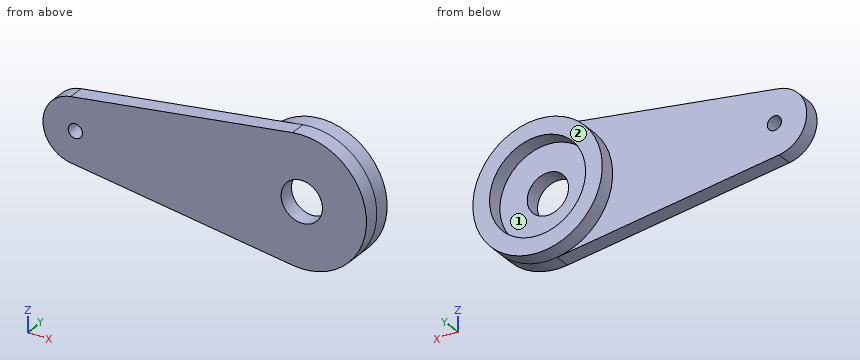
from build123d import *
from build123d.topology import SkipClean

# Parameters (mm, degrees)
EXTRUDE1_DEPTH                      = 6.35
EXTRUDE2_START                      = 6.35
SKETCH2_R                           = 25.4
EXTRUDE2_DEPTH                      = 6.35
F_7_32_0_21875_DIAMETER_HOLE1_D     = 5.55625
F_7_32_0_21875_DIAMETER_HOLE1_DEPTH = 25.4
F_7_32_0_21875_DIAMETER_HOLE1_TIP   = 1.669265907
SKETCH5_R                           = 18.848677946
EXTRUDE3_DEPTH                      = 6.35
SKETCH6_R                           = 8.113502116
EXTRUDE5_DEPTH                      = 118.260276735


with BuildPart() as part:
    # Sketch1 → Extrude1 (new body)
    with BuildSketch(Plane(origin=(0, 0, 0), x_dir=(1, 0, 0), z_dir=(0, 1, 0))):
        with BuildLine():
            Line((-1.814285714, 12.569740146), (85.271428571, 25.139480293))
            ThreePointArc((85.271428571, 25.139480293), (114.3, 0), (85.271428571, -25.139480293))
            Line((85.271428571, -25.139480293), (-1.814285714, -12.569740146))
            ThreePointArc((-1.814285714, -12.569740146), (-12.7, 0), (-1.814285714, 12.569740146))
        make_face()
    extrude(amount=-EXTRUDE1_DEPTH)

    # Sketch2 → Extrude2 (add)
    with SkipClean():  # the faces are left unmerged after this step: merging them gives an invalid solid
        with BuildSketch(Plane(origin=(0, 0, 0), x_dir=(1, 0, 0), z_dir=(0, 1, 0)).offset(EXTRUDE2_START)):
            with Locations(Location((88.9, 0, 0), (0, 0, 270))):
                Circle(SKETCH2_R)
        extrude(amount=-EXTRUDE2_DEPTH)

    # 7/32 (0.21875) Diameter Hole1
    with Locations(Plane.ZX):
        with Locations((0, 0)):
            Hole(F_7_32_0_21875_DIAMETER_HOLE1_D / 2, depth=F_7_32_0_21875_DIAMETER_HOLE1_DEPTH)
            with Locations((0, 0, -(F_7_32_0_21875_DIAMETER_HOLE1_DEPTH + F_7_32_0_21875_DIAMETER_HOLE1_TIP / 2))):  # 118° drill point
                Cone(0, F_7_32_0_21875_DIAMETER_HOLE1_D / 2, F_7_32_0_21875_DIAMETER_HOLE1_TIP, mode=Mode.SUBTRACT)

    # Sketch5 → Extrude3 (cut)
    with SkipClean():  # the faces are left unmerged after this step: merging them gives an invalid solid
        with BuildSketch(Plane(origin=(0, 6.35, 0), x_dir=(-1, 0, 0), z_dir=(0, 1, 0))):
            with Locations(Location((-88.9, 0, 0), (0, 0, 90))):
                Circle(SKETCH5_R)
        extrude(amount=-EXTRUDE3_DEPTH, mode=Mode.SUBTRACT)

    # Sketch6 → Extrude5 (cut, through all)
    with SkipClean():  # the faces are left unmerged after this step: merging them gives an invalid solid
        with BuildSketch(Plane(origin=(0, 0, 0), x_dir=(-1, 0, 0), z_dir=(0, 1, 0))):
            with Locations(Location((-88.9, 0, 0), (0, 0, 90))):
                Circle(SKETCH6_R)
        extrude(amount=-EXTRUDE5_DEPTH, mode=Mode.SUBTRACT)


solid = part.part
Input: part model. Units: mm. Frame: model coordinates. Face numbers are marked on the shaded views. Give positions to 0.01 mm unless a question says otherwise; leave off trailing zeros. Order: outer loops, then holes, each group sorted by start corner. A loop starts at its lowest first (then second) coordinate and runs counter-clockwise, first axis right, second up. Notation, with made-up numbers: M 44.5,22 L 98.5,22 A11 cw 98.5,38 Z; hole C -40,19 d4. An arc over 180 degrees is marked long. Answer as a JSON object with one key per item and string values.
1. Cut plane C-C, the plane y = -1.25. Output: boundary loops of the cut face in (x, z).
Result sheet:
{"outline": "M -1.81,-12.57 L 85.27,-25.14 A25.4 ccw long 85.27,25.14 L -1.81,12.57 A12.7 ccw Z; hole C 0,0 d5.56; hole C 88.9,0 d16.23"}
2. Cut plane D-D, the plane y = 4.5. Output: boundary loops of the cut face in (x, z), and give its area (3 significant figures).
Result sheet:
{"outline": "C 88.9,0 d50.8; hole C 88.9,0 d37.7", "area": "911 mm²"}
3. Cut plane B-B, the plane x = 88.9. Output: boundary loops of the cut face in (y, z).
Result sheet:
{"outline": "M -6.35,-25.4 L 6.35,-25.4 L 6.35,-18.85 L 0,-18.85 L 0,-8.11 L -6.35,-8.11 Z; M -6.35,8.11 L 0,8.11 L 0,18.85 L 6.35,18.85 L 6.35,25.4 L -6.35,25.4 Z"}
4. Ray query, line 1 (X direction, y = -1.75, z = 0); line 2 (X direction, y = 2, z = 0); line 3 (Y direction, x = 63, z = -17). Return the intervals inside material, ascending. Write a range as [from, to].
Result sheet:
{"line 1": "[-12.7, -2.78], [2.78, 80.79], [97.01, 114.3]", "line 2": "[63.5, 70.05], [107.75, 114.3]", "line 3": "[-6.35, 0]"}
5. Cut plane A-A, the plane z = 0. Output: boundary loops of the cut face in (x, y), and give its area (3 significant figures).
Result sheet:
{"outline": "M -12.7,-6.35 L -2.78,-6.35 L -2.78,0 L -12.7,0 Z; M 2.78,-6.35 L 80.79,-6.35 L 80.79,0 L 70.05,0 L 70.05,6.35 L 63.5,6.35 L 63.5,0 L 2.78,0 Z; M 97.01,-6.35 L 114.3,-6.35 L 114.3,6.35 L 107.75,6.35 L 107.75,0 L 97.01,0 Z", "area": "751 mm²"}
6. First-contact query: P1, Ø1, axis at x = 67, y = -3, coming from the -Z side; P2, Ø7, axis at x = 0, z = 0, coming from the +Y side; P3, Ø4, axis at x = 3, y = -3.5, coming from the -Z side. Flat tips, straight axial feed; report the tip coordinate or a pass-through.
Result sheet:
{"P1": "z = -22.57", "P2": "y = 0", "P3": "z = -13.55"}
7. Pull-direction query (X, two-part tool) for the marked faces 1 and 2; classes: +X half, -X half, draft (parallel to the pull), parting line (faces both ways), or undercut.
Result sheet:
{"face 1": "undercut", "face 2": "draft"}
